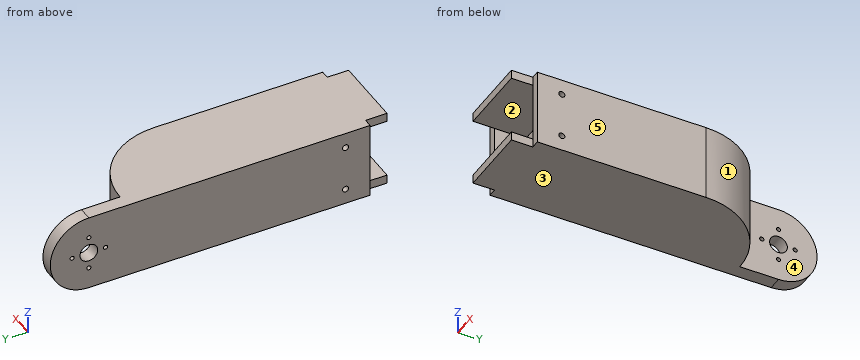
```python
from build123d import *

# Parameters (mm, degrees)
SKETCH1_W               = 50
SKETCH1_H               = 150
BOSS_EXTRUDE1_DEPTH     = 55
CUT_EXTRUDE1_DEPTH      = 168.406690428
CUT_EXTRUDE1_DEPTH_BACK = 45
SKETCH2_R               = 10.25
SKETCH7_R               = 1
SKETCH7_R_2             = 4.25
CUT_EXTRUDE3_DEPTH      = 10
SKETCH8_W               = 55
SKETCH8_H               = 55
SKETCH8_R               = 10.25
BOSS_EXTRUDE2_DEPTH     = 50
SKETCH10_W              = 8
SKETCH10_H              = 10.25
SKETCH10_W_2            = 17
SKETCH10_H_2            = 1
SKETCH10_W_3            = 34
SKETCH10_H_3            = 20
SKETCH10_H_4            = 5
CUT_EXTRUDE4_DEPTH      = 214.717102732
SKETCH11_W              = 34
SKETCH11_H              = 13.25
BOSS_EXTRUDE4_DEPTH     = 25
SKETCH13_W              = 55
SKETCH13_H              = 10
CUT_EXTRUDE5_DEPTH      = 8
SKETCH14_R              = 5.030159043
CUT_EXTRUDE6_DEPTH      = 8
SKETCH15_W              = 34
SKETCH15_H              = 0.25
BOSS_EXTRUDE5_DEPTH     = 13.25
CUT_EXTRUDE7_DEPTH      = 181.416185527
BOSS_EXTRUDE6_START     = 1.5
SKETCH19_R              = 10.25
SKETCH19_R_2            = 1
SKETCH19_R_3            = 4.25
BOSS_EXTRUDE6_DEPTH     = 1.5
CUT_EXTRUDE8_DEPTH      = 184.89467094
SKETCH21_R              = 5.030159043
SKETCH21_R_2            = 4.5
BOSS_EXTRUDE7_DEPTH     = 8
SKETCH24_W              = 4
SKETCH24_H              = 30
CUT_EXTRUDE10_DEPTH     = 181.416185527
SKETCH25_W              = 55
SKETCH25_H              = 86.25
CUT_EXTRUDE11_DEPTH     = 4
BOSS_EXTRUDE8_START     = 4
SKETCH26_R              = 1
SKETCH26_R_2            = 4.25
BOSS_EXTRUDE8_DEPTH     = 4
SKETCH27_W              = 4
SKETCH27_H              = 123.25
CUT_EXTRUDE12_DEPTH     = 181.416185527
CUT_EXTRUDE13_DEPTH     = 180.905530765
SKETCH29_W              = 42
SKETCH29_H              = 9
CUT_EXTRUDE15_DEPTH     = 174.776436838
SKETCH30_R              = 4.5
SKETCH30_R_2            = 1.45
BOSS_EXTRUDE9_DEPTH     = 4


with BuildPart() as part:
    # Sketch1 → Boss-Extrude1 (new body)
    with BuildSketch(Plane.XY):
        with Locations((0, -75)):
            Rectangle(SKETCH1_W, SKETCH1_H)
    extrude(amount=-BOSS_EXTRUDE1_DEPTH)

    # Sketch2 → Cut-Extrude1 (cut, two sides: drawn at the far end of the back side and taken through both)
    with BuildSketch(Plane(origin=(25, 0, 0), x_dir=(0, 0, -1), z_dir=(1, 0, 0)).offset(-CUT_EXTRUDE1_DEPTH_BACK)):
        with Locations(Location((27.5, -25, 0), (0, 0, 270))):
            Circle(SKETCH2_R)
    extrude(amount=CUT_EXTRUDE1_DEPTH + CUT_EXTRUDE1_DEPTH_BACK, mode=Mode.SUBTRACT)

    # Sketch7 → Cut-Extrude3 (cut)
    with BuildSketch(Plane(origin=(-20, 0, 0), x_dir=(0, 0, -1), z_dir=(1, 0, 0))):
        with Locations(Location((27.5, -17, 0), (0, 0, 90))):
            Circle(SKETCH7_R)
        with Locations(Location((35.5, -25, 0), (0, 0, 90))):
            Circle(SKETCH7_R)
        with Locations(Location((27.5, -33, 0), (0, 0, 90))):
            Circle(SKETCH7_R)
        with Locations(Location((19.5, -25, 0), (0, 0, 90))):
            Circle(SKETCH7_R)
        with Locations(Location((27.5, -25, 0), (0, 0, 90))):
            Circle(SKETCH7_R_2)
    extrude(amount=-CUT_EXTRUDE3_DEPTH, mode=Mode.SUBTRACT)

    # Sketch8 → Boss-Extrude2 (add)
    with BuildSketch(Plane(origin=(25, 0, 0), x_dir=(0, 0, -1), z_dir=(1, 0, 0))):
        with Locations((27.5, -177.5)):
            Rectangle(SKETCH8_W, SKETCH8_H)
        with Locations(Location((27.5, -180, 0), (0, 0, 90))):
            Circle(SKETCH8_R, mode=Mode.SUBTRACT)
    extrude(amount=-BOSS_EXTRUDE2_DEPTH)

    # Sketch10 → Cut-Extrude4 (cut, through all)
    with BuildSketch(Plane.XY):
        Polygon((-17, -205), (17, -205), (17, -191.25), (0, -191.25), (-17, -191.25), align=None)
        Polygon((-25, -205), (-17, -205), (-17, -191.25), (-17, -190.25), (-25, -190.25), align=None)
        Polygon((17, -191.25), (17, -205), (25, -205), (25, -190.25), (17, -190.25), align=None)
        with Locations((-21, -185.125)):
            Rectangle(SKETCH10_W, SKETCH10_H)
        with Locations((-21, -174.875)):
            Rectangle(SKETCH10_W, SKETCH10_H)
        with Locations((21, -174.875)):
            Rectangle(SKETCH10_W, SKETCH10_H)
        with Locations((21, -185.125)):
            Rectangle(SKETCH10_W, SKETCH10_H)
        with Locations((-8.5, -185.125)):
            Rectangle(SKETCH10_W_2, SKETCH10_H)
        with Locations((8.5, -185.125)):
            Rectangle(SKETCH10_W_2, SKETCH10_H)
        Polygon((0, -180), (17, -180), (17, -169.75), (-17, -169.75), (-17, -180), align=None)
        with Locations((-8.5, -190.75)):
            Rectangle(SKETCH10_W_2, SKETCH10_H_2)
        with Locations((8.5, -190.75)):
            Rectangle(SKETCH10_W_2, SKETCH10_H_2)
        with Locations((0, -154.75)):
            Rectangle(SKETCH10_W_3, SKETCH10_H_3)
        with Locations((0, -167.25)):
            Rectangle(SKETCH10_W_3, SKETCH10_H_4)
    extrude(amount=-CUT_EXTRUDE4_DEPTH, mode=Mode.SUBTRACT)

    # Sketch11 → Boss-Extrude4 (add)
    with BuildSketch(Plane.XZ.offset(144.75)):
        with Locations((0, -6.625)):
            Rectangle(SKETCH11_W, SKETCH11_H)
        with Locations((0, -48.375)):
            Rectangle(SKETCH11_W, SKETCH11_H)
    extrude(amount=BOSS_EXTRUDE4_DEPTH)

    # Sketch13 → Cut-Extrude5 (cut)
    with BuildSketch(Plane(origin=(25, 0, 0), x_dir=(0, 0, -1), z_dir=(1, 0, 0))):
        with Locations((27.5, -164.75)):
            Rectangle(SKETCH13_W, SKETCH13_H)
    cut_extrude5 = extrude(amount=-CUT_EXTRUDE5_DEPTH, mode=Mode.SUBTRACT)

    # Mirror2: Cut-Extrude5 across plane
    add(cut_extrude5.mirror(Plane(origin=(0, 0, 0), x_dir=(0, 0, 1), z_dir=(1, 0, 0))), mode=Mode.SUBTRACT)

    # Sketch14 → Cut-Extrude6 (cut)
    with BuildSketch(Plane(origin=(25, 0, 0), x_dir=(0, 0, -1), z_dir=(1, 0, 0))):
        with Locations(Location((16.5, -148, 0), (0, 0, 90))):
            Circle(SKETCH14_R)
        with Locations(Location((38.5, -148, 0), (0, 0, 90))):
            Circle(SKETCH14_R)
    cut_extrude6 = extrude(amount=-CUT_EXTRUDE6_DEPTH, mode=Mode.SUBTRACT)

    # Mirror3: Cut-Extrude6 across plane
    add(cut_extrude6.mirror(Plane(origin=(0, 0, 0), x_dir=(0, 0, 1), z_dir=(1, 0, 0))), mode=Mode.SUBTRACT)

    # Sketch15 → Boss-Extrude5 (add)
    with BuildSketch(Plane.XY):
        with Locations((0, -169.875)):
            Rectangle(SKETCH15_W, SKETCH15_H)
    boss_extrude5 = extrude(amount=-BOSS_EXTRUDE5_DEPTH)

    # Mirror4: Boss-Extrude5 across plane
    add(boss_extrude5.mirror(Plane.XY.offset(-27.5)))

    # Sketch16 → Cut-Extrude7 (cut, through all)
    with BuildSketch(Plane.XY):
        Polygon((-18.5, 0), (-18.5, -14.75), (-18.5, -35.25), (-18.5, -43.5), (25, -43.5), (25, 0), align=None)
    extrude(amount=-CUT_EXTRUDE7_DEPTH, mode=Mode.SUBTRACT)

    # Sketch19 → Boss-Extrude6 (add)
    with BuildSketch(Plane(origin=(-20, 0, 0), x_dir=(0, 0, -1), z_dir=(1, 0, 0)).offset(BOSS_EXTRUDE6_START)):
        with Locations((27.5, -25)):
            Circle(SKETCH19_R)
        with Locations(Location((27.5, -17, 0), (0, 0, 90))):
            Circle(SKETCH19_R_2, mode=Mode.SUBTRACT)
        with Locations(Location((27.5, -33, 0), (0, 0, 90))):
            Circle(SKETCH19_R_2, mode=Mode.SUBTRACT)
        with Locations(Location((19.5, -25, 0), (0, 0, 90))):
            Circle(SKETCH19_R_2, mode=Mode.SUBTRACT)
        with Locations(Location((35.5, -25, 0), (0, 0, 90))):
            Circle(SKETCH19_R_2, mode=Mode.SUBTRACT)
        with Locations(Location((27.5, -25, 0), (0, 0, 90))):
            Circle(SKETCH19_R_3, mode=Mode.SUBTRACT)
    extrude(amount=-BOSS_EXTRUDE6_DEPTH)

    # Sketch20 → Cut-Extrude8 (cut, through all)
    with BuildSketch(Plane(origin=(-18.5, 0, 0), x_dir=(0, 0, -1), z_dir=(1, 0, 0))):
        with BuildLine():
            Line((0, 0), (0, -43.5))
            Line((0, -43.5), (9, -43.5))
            Line((9, -43.5), (9, -25))
            ThreePointArc((9, -25), (27.5, -6.5), (46, -25))
            Line((46, -25), (46, -43.5))
            Line((46, -43.5), (55, -43.5))
            Line((55, -43.5), (55, 0))
            Line((55, 0), (0, 0))
        make_face()
    extrude(amount=-CUT_EXTRUDE8_DEPTH, mode=Mode.SUBTRACT)

    # Sketch21 → Boss-Extrude7 (add)
    # profile 1 of 2: a face of its own
    with BuildSketch(Plane(origin=(25, 0, 0), x_dir=(0, 0, -1), z_dir=(1, 0, 0))):
        with Locations(Location((16.5, -148, 0), (0, 0, 229.751587581))):
            Circle(SKETCH21_R)
        with Locations(Location((16.5, -148, 0), (0, 0, 90))):
            Circle(SKETCH21_R_2, mode=Mode.SUBTRACT)
    # profile 2 of 2: a face of its own
    with BuildSketch(Plane(origin=(25, 0, 0), x_dir=(0, 0, -1), z_dir=(1, 0, 0))):
        with Locations(Location((38.5, -148, 0), (0, 0, 310.248412419))):
            Circle(SKETCH21_R)
        with Locations(Location((38.5, -148, 0), (0, 0, 90))):
            Circle(SKETCH21_R_2, mode=Mode.SUBTRACT)
    boss_extrude7 = extrude(amount=-BOSS_EXTRUDE7_DEPTH)

    # Mirror5: Boss-Extrude7 across plane
    add(boss_extrude7.mirror(Plane(origin=(0, 0, 0), x_dir=(0, 0, 1), z_dir=(1, 0, 0))))

    # Sketch24 → Cut-Extrude10 (cut, through all)
    with BuildSketch(Plane.XY):
        with Locations((-23, -144.75)):
            Rectangle(SKETCH24_W, SKETCH24_H)
        with Locations((23, -144.75)):
            Rectangle(SKETCH24_W, SKETCH24_H)
    extrude(amount=-CUT_EXTRUDE10_DEPTH, mode=Mode.SUBTRACT)

    # Sketch25 → Cut-Extrude11 (cut)
    with BuildSketch(Plane(origin=(25, 0, 0), x_dir=(0, 0, -1), z_dir=(1, 0, 0))):
        with Locations((27.5, -86.625)):
            Rectangle(SKETCH25_W, SKETCH25_H)
    extrude(amount=-CUT_EXTRUDE11_DEPTH, mode=Mode.SUBTRACT)

    # Sketch26 → Boss-Extrude8 (add)
    with BuildSketch(Plane(origin=(-18.5, 0, 0), x_dir=(0, 0, -1), z_dir=(1, 0, 0)).offset(BOSS_EXTRUDE8_START)):
        with BuildLine():
            Line((46, -43.5), (46, -25))
            ThreePointArc((46, -25), (27.5, -6.5), (9, -25))
            Line((9, -25), (9, -43.5))
            Line((9, -43.5), (46, -43.5))
        make_face()
        with Locations(Location((35.5, -25, 0), (0, 0, 90))):
            Circle(SKETCH26_R, mode=Mode.SUBTRACT)
        with Locations(Location((27.5, -25, 0), (0, 0, 90))):
            Circle(SKETCH26_R_2, mode=Mode.SUBTRACT)
        with Locations(Location((19.5, -25, 0), (0, 0, 90))):
            Circle(SKETCH26_R, mode=Mode.SUBTRACT)
        with Locations(Location((27.5, -33, 0), (0, 0, 90))):
            Circle(SKETCH26_R, mode=Mode.SUBTRACT)
        with Locations(Location((27.5, -17, 0), (0, 0, 90))):
            Circle(SKETCH26_R, mode=Mode.SUBTRACT)
    extrude(amount=-BOSS_EXTRUDE8_DEPTH)

    # Sketch27 → Cut-Extrude12 (cut, through all)
    with BuildSketch(Plane.XY):
        with Locations((-23, -68.125)):
            Rectangle(SKETCH27_W, SKETCH27_H)
    extrude(amount=-CUT_EXTRUDE12_DEPTH, mode=Mode.SUBTRACT)

    # Sketch28 → Cut-Extrude13 (cut, through all)
    with BuildSketch(Plane.XY):
        with BuildLine():
            Line((21, -43.5), (-14.5, -43.5))
            ThreePointArc((-14.5, -43.5), (10.602290732, -53.897709268), (21, -79))
            Line((21, -79), (21, -43.5))
        make_face()
    extrude(amount=-CUT_EXTRUDE13_DEPTH, mode=Mode.SUBTRACT)

    # Sketch29 → Cut-Extrude15 (cut, through all)
    with BuildSketch(Plane.XZ.offset(170)):
        with Locations((0, -50.5)):
            Rectangle(SKETCH29_W, SKETCH29_H)
        with Locations((0, -4.5)):
            Rectangle(SKETCH29_W, SKETCH29_H)
    extrude(amount=-CUT_EXTRUDE15_DEPTH, mode=Mode.SUBTRACT)

    # Sketch30 → Boss-Extrude9 (add)
    # profile 1 of 2: a face of its own
    with BuildSketch(Plane(origin=(21, 0, 0), x_dir=(0, 0, -1), z_dir=(1, 0, 0))):
        with Locations(Location((16.5, -148, 0), (0, 0, 223.761742693))):
            Circle(SKETCH30_R)
        with Locations((16.5, -148)):
            Circle(SKETCH30_R_2, mode=Mode.SUBTRACT)
    # profile 2 of 2: a face of its own
    with BuildSketch(Plane(origin=(21, 0, 0), x_dir=(0, 0, -1), z_dir=(1, 0, 0))):
        with Locations(Location((38.5, -148, 0), (0, 0, 316.238257307))):
            Circle(SKETCH30_R)
        with Locations((38.5, -148)):
            Circle(SKETCH30_R_2, mode=Mode.SUBTRACT)
    boss_extrude9 = extrude(amount=-BOSS_EXTRUDE9_DEPTH)

    # Mirror6: Boss-Extrude9 across plane
    add(boss_extrude9.mirror(Plane(origin=(0, 0, 0), x_dir=(0, 0, 1), z_dir=(1, 0, 0))))


solid = part.part
```
Model file for the job. Use its own axes, mm. Face numbers are marked on the shaded views. A direction names the side the tool comes from. Coordinates: 2 decimals unless noted, no trailing zeros. Order: outer loops, then holes, each group sorted by start corner. A loop starts at its lowest first (then second) coordinate and runs counter-clockwise, first axis right, second up. Notation, with made-up numbers: M 68.5,15.5 L 103.5,15.5 A26 cw 103.5,48.5 Z; hole C -39,41.5 d1. An arc over 180 degrees is marked long. Answer as CSV lines item,"result".
(1) Band-saw the part on C-C, the plane x = 10. List the corners of the cut face in (y, z), then the cut area to 3 significant figures.
Geometry says:
outline,"M -170,-46 L -53.31,-46 L -53.31,-9 L -170,-9 L -170,-13.25 L -144.75,-13.25 L -144.75,-41.75 L -170,-41.75 Z"
area,"3,600 mm2"
(2) 3-axis set-ups, long thin cutter, end or side, ignore diameter. For the marked faces 4 and 5: which of +Z, -Z, +X, -X, +Y, -Y reach the whole face in a straight line?
Geometry says:
face 4,"+Z, -Z, +X, +Y"
face 5,"+Z, -Z, +X, +Y, -Y"
(3) Band-saw the part on A-A, the plane y = -148. List the corners of the cut face in (x, z).
Geometry says:
outline,"M -21,-46 L 21,-46 L 21,-39.95 L 17,-39.95 L 17,-41.75 L -17,-41.75 L -17,-39.95 L -21,-39.95 Z; M -21,-37.05 L -17,-37.05 L -17,-17.95 L -21,-17.95 Z; M -21,-15.05 L -17,-15.05 L -17,-13.25 L 17,-13.25 L 17,-15.05 L 21,-15.05 L 21,-9 L -21,-9 Z; M 17,-37.05 L 21,-37.05 L 21,-17.95 L 17,-17.95 Z"
(4) Flat gauge pins, fed straight in: pin 1 (6 mm diameter, centred on x = -1, z = -17, fed in from -Y); pin 2 (10 mm diameter, centred on y = -25, z = -27.5, fed in from +X); pin 3 (6 mm diameter, centred on x = 10.5, z = -21.5, fed in from +Y). Where does each tip first touch, or does it go through?
Geometry says:
pin 1,"stops at y = -144.75"
pin 2,"stops at x = -14.5"
pin 3,"stops at y = -51.14"
(5) Band-saw the part on B-B, the plane z = -16.5. List the corners of the cut face in (x, y), then the cut area to 3 significant figures.
Geometry says:
outline,"M -21,-159.75 L -17,-159.75 L -17,-149.45 L -21,-149.45 Z; M -21,-146.55 L -17,-146.55 L -17,-144.75 L 17,-144.75 L 17,-146.55 L 21,-146.55 L 21,-79 A35.5 ccw -14.5,-43.5 L -14.5,-10.13 L -21,-10.13 Z; M 17,-159.75 L 21,-159.75 L 21,-149.45 L 17,-149.45 Z"
area,"4,300 mm2"
(6) Wall check: line 1 along Z through (x, y) = (-19, -148); line 2 along Z through (x, y) = (-19, -25); line 3 along X through (y, z) = (-153, -37). Give the ranges that are in metal, low to high.
Geometry says:
line 1,"z = -46 to -39.95, -37.05 to -17.95, -15.05 to -9"
line 2,"z = -46 to -36.5, -34.5 to -31.75, -23.25 to -20.5, -18.5 to -9"
line 3,"x = -21 to -17, 17 to 21"
(7) Band-saw the part on D-D, the plane z = -25. List the corners of the cut face in (x, y), then the cut area to 3 significant figures.
Geometry says:
outline,"M -21,-159.75 L -17,-159.75 L -17,-144.75 L 17,-144.75 L 17,-159.75 L 21,-159.75 L 21,-79 A35.5 ccw -14.5,-43.5 L -14.5,-28.44 L -21,-28.44 Z; M -21,-21.56 L -14.5,-21.56 L -14.5,-6.67 L -21,-6.67 Z"
area,"4,300 mm2"
(8) Pull direction Z, two halves, no side cores. Call the marked faces 1, 2 and 3: +Z half, -Z half, draft (parallel to the pull), parting line (faces both ways), or undercut.
Geometry says:
face 1,"draft"
face 2,"undercut"
face 3,"-Z half"
